Geometry check sheet. Reference: the model listing, model coordinates, mm. Face numbers are marked on the shaded views. Coordinates: 2 decimals unless noted, no trailing zeros. Write each loop counter-clockwise with the first axis right and the second up, starting at its lowest first coordinate (ties: lowest second). Pieces come first, ordered by that corner, then holes.
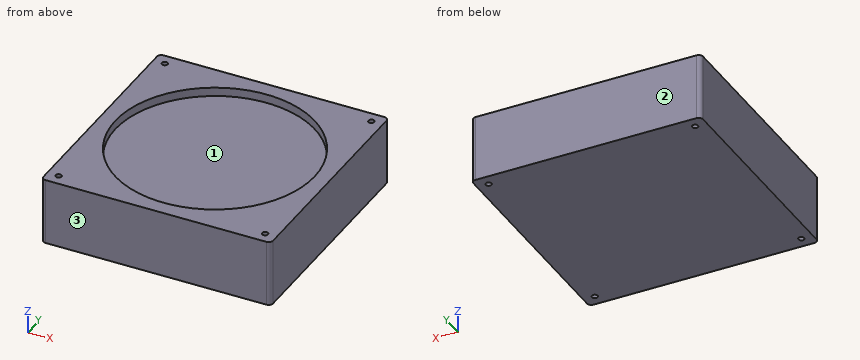
from build123d import *

# Parameters (mm, degrees)
SKETCH1_W             = 132
SKETCH1_H             = 132
BOSS_EXTRUDE1_DEPTH   = 38.29
FILLET1_R             = 2.54
M4X0_7_TAPPED_HOLE1_D = 3.3
SKETCH4_R             = 57.341527379
CUT_EXTRUDE1_DEPTH    = 5.08


with BuildPart() as part:
    # Sketch1 → Boss-Extrude1 (new body)
    with BuildSketch(Plane.XY):
        Rectangle(SKETCH1_W, SKETCH1_H)
    extrude(amount=BOSS_EXTRUDE1_DEPTH)

    # Fillet1
    fillet1_edges = [part.edges().sort_by_distance(p)[0] for p in [
        (66, -66, 19.145),
        (-66, -66, 19.145),
        (-66, 66, 19.145),
        (66, 66, 19.145),
    ]]
    fillet(fillet1_edges, radius=FILLET1_R)

    # M4x0.7 Tapped Hole1 (through all)
    with Locations(Plane.XY.offset(38.29)):
        with Locations((-59.4, 59.4), (59.4, 59.4), (59.4, -59.4), (-59.4, -59.4)):
            Hole(M4X0_7_TAPPED_HOLE1_D / 2)

    # Sketch4 → Cut-Extrude1 (cut)
    with BuildSketch(Plane.XY.offset(38.29)):
        Circle(SKETCH4_R)
    extrude(amount=-CUT_EXTRUDE1_DEPTH, mode=Mode.SUBTRACT)


solid = part.part
1. Thickness scan on line 1 along Y through (x, z) = (59.5, 14.5); line 2 along X through (y, z) = (-58, 2); line 3 along X through (y, z) = (59, 13). Record the ranges inside material, lowest first.
Computed values:
line 1: y = -66 to -61.05, -57.75 to 57.75, 61.05 to 66
line 2: x = -66 to -60.27, -58.53 to 58.53, 60.27 to 66
line 3: x = -66 to -61, -57.8 to 57.8, 61 to 66
2. Sectioned sample at A-A, the plane y = 59.4. Record the boundary of the cut face in (x, z).
Computed values:
outline: (-66, 0) - (-61.05, 0) - (-61.05, 38.29) - (-66, 38.29) - close; (-57.75, 0) - (57.75, 0) - (57.75, 38.29) - (-57.75, 38.29) - close; (61.05, 0) - (66, 0) - (66, 38.29) - (61.05, 38.29) - close
3. Draft check along Y on the marked faces 1, 2 and 3. Enter one of: released by +Y, released by -Y, zero draft, split by the parting line, or undercut.
Computed values:
face 1: undercut
face 2: released by +Y
face 3: released by -Y
4. Sectioned sample at C-C, the plane y = 0. Record the boundary of the cut face in (x, z), and give its area (3 significant figures).
Computed values:
outline: (-66, 0) - (66, 0) - (66, 38.29) - (57.34, 38.29) - (57.34, 33.21) - (-57.34, 33.21) - (-57.34, 38.29) - (-66, 38.29) - close
area: 4,470 mm2
5. Sectioned sample at D-D, the plane x = -10.5. Record the boundary of the cut face in (y, z).
Computed values:
outline: (-66, 0) - (66, 0) - (66, 38.29) - (56.37, 38.29) - (56.37, 33.21) - (-56.37, 33.21) - (-56.37, 38.29) - (-66, 38.29) - close
6. Gauge pin test, flat end, axial feed: pin 1 Ø10 at (x, y) = (16, -12.5) entering from +Z. Record the tip position at first contact, or that the pin passes through.
Computed values:
pin 1: stops at z = 33.21
